Answer from the drawing. Dimensions are ordinates in mm from the lowest x, y and z of the part. A direction names the side the tool comes from. Coordinates: 2 decimals unless noted, no trailing zeros. Write each loop counter-clockwise with the first axis right and the second up, starting at its lowest first coordinate (ties: lowest second). Pieces come first, ordered by that corner, then holes.
(1) Straight lines are drawn through the part: line 1 along Z through (x, y) = (4, 3.85); line 2 along X through (y, z) = (6.5, 8); line 3 along X through (y, z) = (40, 7.75). For each, find the intervals that lie inside material, in ascending order.
(2) The part is cut by section D-D, the plane x = 13. Determine the outline of the cut face in (y, z) (1 decimal), and give its area (3 significant figures).
(3) Given pin 1 (2.5 mm diameter, centred on y = 2.5, z = 4, fed in from +X); pin 2 (5 mm diameter, centred on y = 10, z = 5.5, fed in from -X); pin 3 (2.5 mm diameter, centred on y = 39.5, z = 5.5, fed in from +X); pin 4 (2 mm diameter, centred on y = 3.85, z = 5, fed in from -X), each flat-ended and moving along its own axis, determine where each tip first touches the part or whether it passes through.
(4) Which of the six approach directions +Z, -Z, +X, -X, +Y, -Y give full straight-line access (tool end or side, diameter ignored) to the marked faces 1, 2, 3, 4 and 5?
(5) The part is cut by section B-B, the plane z = 5. State how many separate pieces and enclosed holes the cut face has, and give its area (3 significant figures).
(6) The part is cut by section A-A, the plane y = 3.85. Determine the outline of the cut face in (x, z), and give its area (3 significant figures).
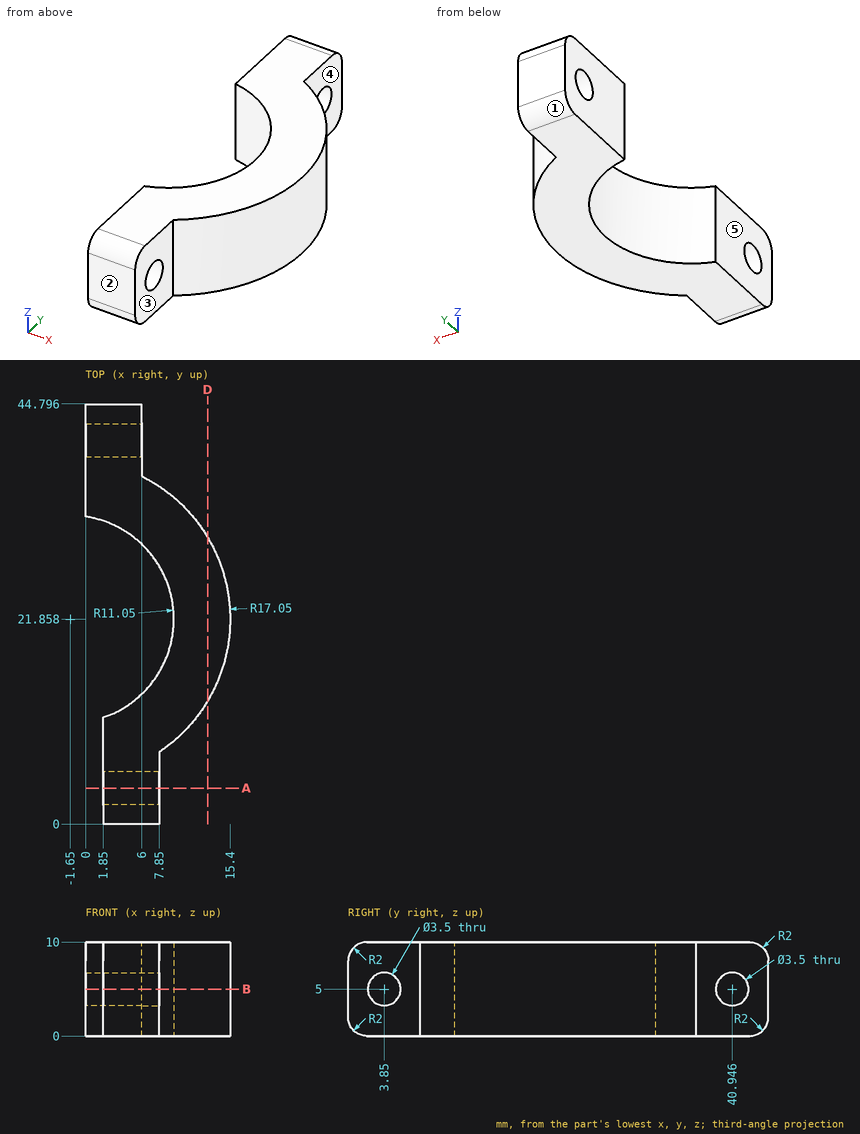
Computed:
1. line 1: z = 0 to 3.25, 6.75 to 10
1. line 2: x = 1.85 to 7.85
1. line 3: x = 0 to 6
2. outline: (13.1, 0) - (30.6, 0) - (30.6, 10) - (13.1, 10) - close
2. area: 174 mm2
3. pin 1: stops at x = 7.85
3. pin 2: stops at x = 1.85
3. pin 3: stops at x = 6
3. pin 4: passes through
4. face 1: -Z, +X, -X, +Y
4. face 2: +Z, -Z, +X, -X, -Y
4. face 3: +Z, -Z, +X, -Y
4. face 4: +Z, -Z, +X, +Y
4. face 5: +Z, -Z, -X, -Y
5. separate pieces: 3
5. enclosed holes: 0
5. area: 269 mm2
6. outline: (1.85, 0) - (7.85, 0) - (7.85, 3.25) - (1.85, 3.25) - close; (1.85, 6.75) - (7.85, 6.75) - (7.85, 10) - (1.85, 10) - close
6. area: 39.0 mm2
